Geometry check sheet. Reference: the model listing, model coordinates, mm. Face numbers are marked on the shaded views. A direction names the side the tool comes from. Round coordinates to 2 decimals unless told otherwise and drop trailing zeros. Order: outer loops, then holes, each group sorted by start corner. A loop starts at its lowest first (then second) coordinate and runs counter-clockwise, first axis right, second up. Notation, with made-up numbers: (10.5, 39) - (61.5, 39) arc R20 ccw to (61.5, 68) - close; hole circle Ø9 at (11, -25.5). An arc over 180 degrees is marked (long way). Use a Markdown table: item, result. Add a question column.
(1) Mould release check, pull along X, two halves, no side actions. Record for the marked faces 1, 2, 3 and 4: released by +X, released by -X, zero draft, split by the parting line, or undercut.
(2) Section check A-A on y = 48.75. Record the boundary of the cut face in (x, z).
(3) Section check B-B on x = -125.25. Record the boundary of the cut face in (y, z), then the cut area to 3 significant figures.
(4) Thickness scan on line 1 along X through (y, z) = (50, 2.6); line 2 along X through (y, z) = (35, 2.8); line 3 along Y through (x, z) = (-115.75, 1.5). Record the ranges inside material, lowest first. Write a range as [from, to].
(5) Section check D-D on x = -132.5. Record the boundary of the cut face in (y, z), then the cut area to 3 significant figures.
(6) Section check C-C on z = 2.4. Give the number of separate pieces and of enclosed holes in the cut face, then the cut area to 3 significant figures.
(7) Gauge pin test, flat ends, axial feed: P1, Ø0.9, axis at y = 48, z = 1, coming from the -X side; P2, Ø0.9, axis at x = -125, z = 2, coming from the +Y side; P3, Ø2, axis at x = -126, y = 43, coming from the -Z side; P4, Ø1.5, axis at y = 44, z = 1.5, coming from the +X side. Record the tip position at first contact, or that the pin passes through.
(8) Access from +Z, -Z, +X, -X, +Y, -Y to the whole of each face (thin tool, end or side, straight path). Record for the marked faces 5, 6, 7, 8 and 9.
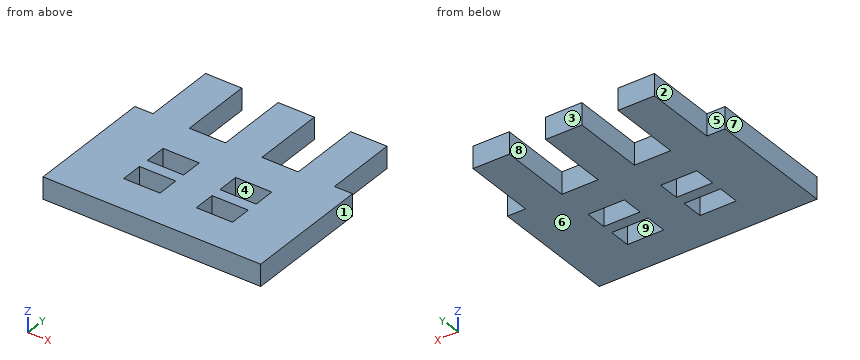
```python
from build123d import *

# Parameters (mm, degrees)
ESQUISSE1_W        = 5
ESQUISSE1_H        = 3
BOSS_EXTRU_1_DEPTH = 3
ESQUISSE2_W        = 2.5
ESQUISSE2_H        = 7.5
BOSS_EXTRU_2_DEPTH = 3


with BuildPart() as part:
    # Esquisse1 → Boss.-Extru.1 (new body)
    with BuildSketch(Plane.XY):
        Polygon((-117.151475887, 41.372526747), (-117.151475887, 51.372526747), (-122.151475887, 51.372526747), (-122.151475887, 41.372526747), (-127.151475887, 41.372526747), (-127.151475887, 51.372526747), (-132.151475887, 51.372526747), (-132.151475887, 41.372526747), (-134.651475887, 41.372526747), (-134.651475887, 36.372526747), (-132.151475887, 36.372526747), (-132.151475887, 33.372526747), (-134.651475887, 33.372526747), (-134.651475887, 31.872526747), (-132.151475887, 31.872526747), (-132.151475887, 28.872526747), (-134.651475887, 28.872526747), (-134.651475887, 23.872526747), (-104.651475887, 23.872526747), (-104.651475887, 28.872526747), (-107.151475887, 28.872526747), (-107.151475887, 31.872526747), (-104.651475887, 31.872526747), (-104.651475887, 33.372526747), (-107.151475887, 33.372526747), (-107.151475887, 36.372526747), (-104.651475887, 36.372526747), (-104.651475887, 41.372526747), (-107.151475887, 41.372526747), (-107.151475887, 51.372526747), (-112.151475887, 51.372526747), (-112.151475887, 41.372526747), align=None)
        with Locations((-114.651475887, 30.372526747)):
            Rectangle(ESQUISSE1_W, ESQUISSE1_H, mode=Mode.SUBTRACT)
        with Locations((-124.651475887, 30.372526747)):
            Rectangle(ESQUISSE1_W, ESQUISSE1_H, mode=Mode.SUBTRACT)
        with Locations((-114.651475887, 34.872526747)):
            Rectangle(ESQUISSE1_W, ESQUISSE1_H, mode=Mode.SUBTRACT)
        with Locations((-124.651475887, 34.872526747)):
            Rectangle(ESQUISSE1_W, ESQUISSE1_H, mode=Mode.SUBTRACT)
    extrude(amount=BOSS_EXTRU_1_DEPTH)

    # Esquisse2 → Boss.-Extru.2 (add)
    with BuildSketch(Plane(origin=(0, 0, 0), x_dir=(-1, 0, 0), z_dir=(0, 0, -1))):
        with Locations((133.401475887, 32.622526747)):
            Rectangle(ESQUISSE2_W, ESQUISSE2_H)
        with Locations((105.901475887, 32.622526747)):
            Rectangle(ESQUISSE2_W, ESQUISSE2_H)
    extrude(amount=-BOSS_EXTRU_2_DEPTH)


solid = part.part
```
Check sheet entries:
| question | item | result |
|---|---|---|
| 1 | face 1 | released by +X |
| 1 | face 2 | released by -X |
| 1 | face 3 | zero draft |
| 1 | face 4 | undercut |
| 2 | outline | (-132.15, 0) - (-127.15, 0) - (-127.15, 3) - (-132.15, 3) - close; (-122.15, 0) - (-117.15, 0) - (-117.15, 3) - (-122.15, 3) - close; (-112.15, 0) - (-107.15, 0) - (-107.15, 3) - (-112.15, 3) - close |
| 3 | outline | (23.87, 0) - (28.87, 0) - (28.87, 3) - (23.87, 3) - close; (31.87, 0) - (33.37, 0) - (33.37, 3) - (31.87, 3) - close; (36.37, 0) - (41.37, 0) - (41.37, 3) - (36.37, 3) - close |
| 3 | area | 34.5 mm2 |
| 4 | line 1 | x = [-132.15, -127.15], [-122.15, -117.15], [-112.15, -107.15] |
| 4 | line 2 | x = [-134.65, -127.15], [-122.15, -117.15], [-112.15, -104.65] |
| 4 | line 3 | y = [23.87, 28.87], [31.87, 33.37], [36.37, 41.37] |
| 5 | outline | (23.87, 0) - (41.37, 0) - (41.37, 3) - (23.87, 3) - close |
| 5 | area | 52.5 mm2 |
| 6 | separate pieces | 1 |
| 6 | enclosed holes | 4 |
| 6 | area | 615 mm2 |
| 7 | P1 | stops at x = -132.15 |
| 7 | P2 | stops at y = 41.37 |
| 7 | P3 | passes through |
| 7 | P4 | stops at x = -107.15 |
| 8 | face 5 | +Z, -Z, -X, +Y |
| 8 | face 6 | -Z, +X, -X, +Y, -Y |
| 8 | face 7 | +Z, -Z, -X, +Y, -Y |
| 8 | face 8 | +Z, -Z, +Y |
| 8 | face 9 | +Z, -Z |
